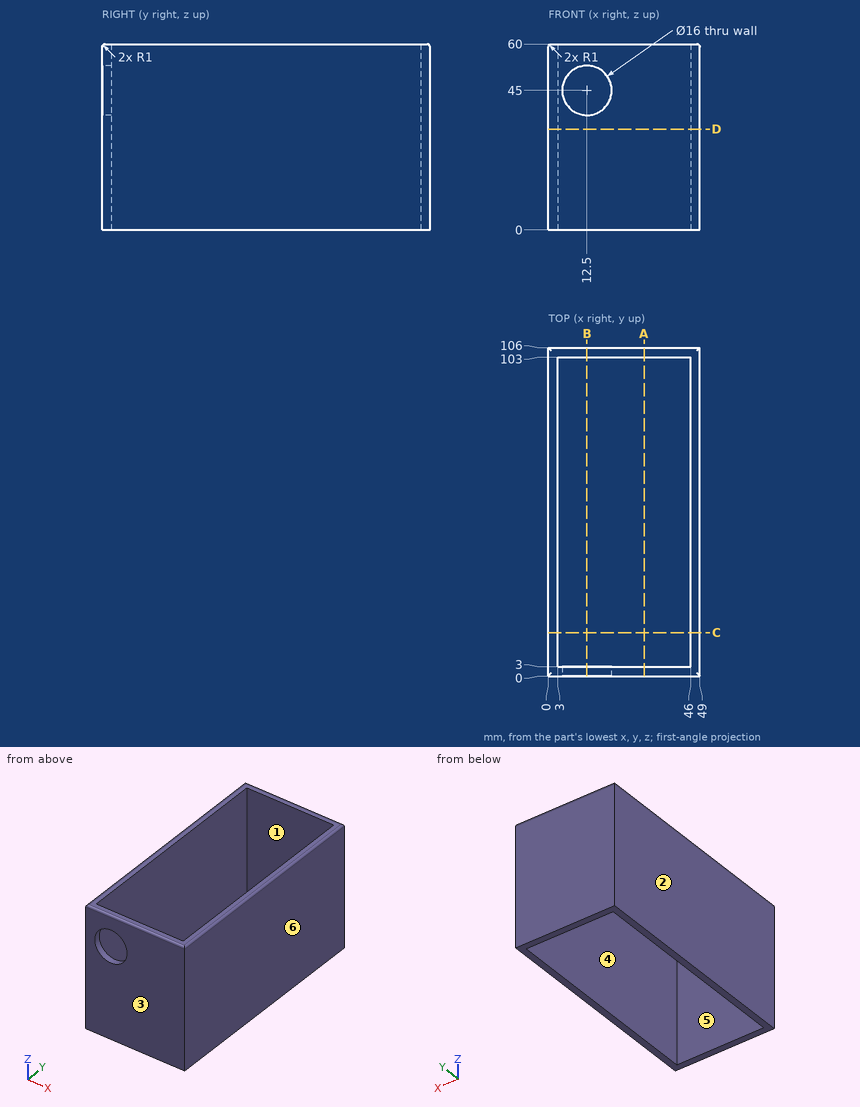
Print and shaded views of the part. All mm, measured from the part's lowest x, y and z. A direction names the side the tool comes from. Round coordinates to 2 decimals unless told otherwise and drop trailing zeros. Write each loop counter-clockwise with the first axis right and the second up, starting at its lowest first coordinate (ties: lowest second). Pieces come first, ordered by that corner, then holes. Notation, with made-up numbers: (18.25, 5.5) -> (37.25, 5.5) arc R11 cw to (37.25, 13.5) -> close; hole circle Ø5 at (0, 14.5). An arc over 180 degrees is marked (long way). Return JSON: item names as keys, results as strings. Group by question number.
Q1. Pin check, flat tip, straight feed: pin 1 (13 mm diameter, centred on x = 12.5, z = 45, fed in from -Y). Stop position of the tip, or through.
Q2. Which spindle directions (+Z, -Z, +X, -X, +Y, -Y) get a long thin tool onto all of the face, cutting with end or side? Do the marked faces 5 and 6. Say none if no direction does.
Q3. Saw through at C-C on y = 14. Write the cut outline in (x, z).
Q4. Saw through at B-B on x = 12.5. Write the cut outline in (y, z), plus the area to 3 significant figures.
Q5. Probe L1, parallel to Y at x = 35, z = 47.5; L2, parallel to X at y = 88, z = 2; L3, parallel to Z at x = 12.5, y = 1.5. List the from-to ranges inside material, lowest first. Write a range as [from, to].
Q6. Mould opens along Y. For the marked faces 1, 2, 3 and 4 say: pulls with the +Y half, pulls with the -Y half, needs draft (parallel to the pull), parting line crosses it, or undercut.
Q7. Saw through at A-A on x = 31. Write the cut outline in (y, z), plus the area to 3 significant figures.
Q8. Saw through at D-D on z = 32.5. Write the cut outline in (x, y), plus the area to 3 significant figures.
Answer:
{
 "1": {"pin 1": "y = 103"},
 "2": {"face 5": "+Z, -Z", "face 6": "+Z, -Z, +X, +Y, -Y"},
 "3": {"outline": "(0, 0) -> (3, 0) -> (3, 60) -> (1, 60) arc R1 ccw to (0, 59) -> close; (46, 0) -> (49, 0) -> (49, 59) arc R1 ccw to (48, 60) -> (46, 60) -> close"},
 "4": {"outline": "(0, 0) -> (3, 0) -> (3, 37) -> (0, 37) -> close; (0, 53) -> (3, 53) -> (3, 60) -> (1, 60) arc R1 ccw to (0, 59) -> close; (103, 0) -> (106, 0) -> (106, 59) arc R1 ccw to (105, 60) -> (103, 60) -> close", "area": "312 mm2"},
 "5": {"L1": "[0, 3], [103, 106]", "L2": "[0, 3], [46, 49]", "L3": "[0, 37], [53, 60]"},
 "6": {"face 1": "undercut", "face 2": "needs draft", "face 3": "pulls with the -Y half", "face 4": "undercut"},
 "7": {"outline": "(0, 0) -> (3, 0) -> (3, 60) -> (1, 60) arc R1 ccw to (0, 59) -> close; (103, 0) -> (106, 0) -> (106, 59) arc R1 ccw to (105, 60) -> (103, 60) -> close", "area": "360 mm2"},
 "8": {"outline": "(0, 0) -> (49, 0) -> (49, 106) -> (0, 106) -> close; hole (3, 3) -> (46, 3) -> (46, 103) -> (3, 103) -> close", "area": "894 mm2"}
}
